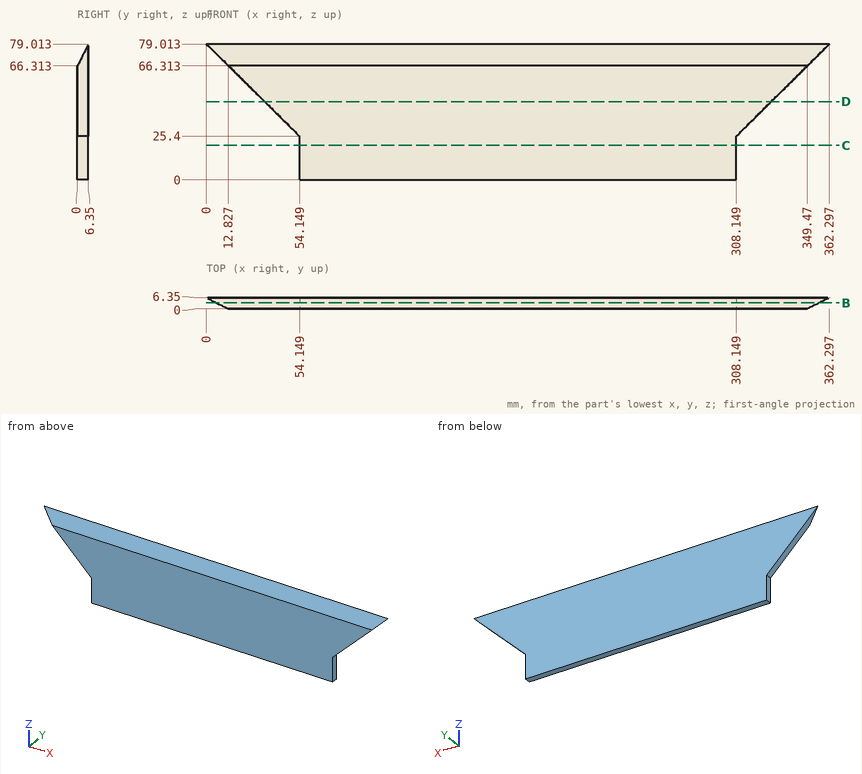
Can you work these out from the drawing? Everything is in mm from the part's minimum corner. Round coordinates to 2 decimals unless told otherwise and drop trailing zeros. Loops run counter-clockwise (first coordinate to the right, second up) from the corner with the lowest first, then second, coordinate; pieces in that order, holes last. Notation, with made-up numbers: (-34, 73.25) - (13, 73.25) arc R21 cw to (13, 97.25) - close; hole circle Ø11 at (71.5, 66). An arc over 180 degrees is marked (long way). Answer in a Markdown table with one row per item. Add a question column.
(1) If we section it at B-B (y = 3.5): Please give me the cut outline in (x, z).
(2) If we section it at D-D (z = 45.5): Please give me the cut outline in (x, y), plus the area to 3 significant figures.
(3) If we section it at C-C (z = 20): Please give me the cut outline in (x, y), plus the area to 3 significant figures.
(4) I'm going to push flat-ended pins straight in: pin 1 (2 mm diameter, centred on x = 305.5, y = 4.5, fed in from +Z) (1 decimal); pin 2 (1 mm diameter, centred on y = 3.5, z = 48.5, fed in from -X). Where does each tip first touch, or does it pass through?
(5) I need wall thicknesses on line 1 along X through (y, z) = (2.5, 19.5); line 2 along X through (y, z) = (5.5, 28) (1 decimal); line 3 along Z through (x, y) = (96.5, 0.75) (1 decimal). Which ranges of each line are inside material? Lowest first, please.
Model answer:
| question | item | result |
|---|---|---|
| 1 | outline | (5.76, 73.31) - (54.15, 25.4) - (54.15, 0) - (308.15, 0) - (308.15, 25.4) - (356.54, 73.31) - close |
| 2 | outline | (33.85, 0) - (328.45, 0) - (328.45, 6.35) - (33.85, 6.35) - close |
| 2 | area | 1,870 mm² |
| 3 | outline | (54.15, 0) - (308.15, 0) - (308.15, 6.35) - (54.15, 6.35) - close |
| 3 | area | 1,610 mm² |
| 4 | pin 1 | stops at z = 77.3 |
| 4 | pin 2 | stops at x = 30.31 |
| 5 | line 1 | x = 54.15 to 308.15 |
| 5 | line 2 | x = 51.5 to 310.8 |
| 5 | line 3 | z = 0 to 67.8 |
